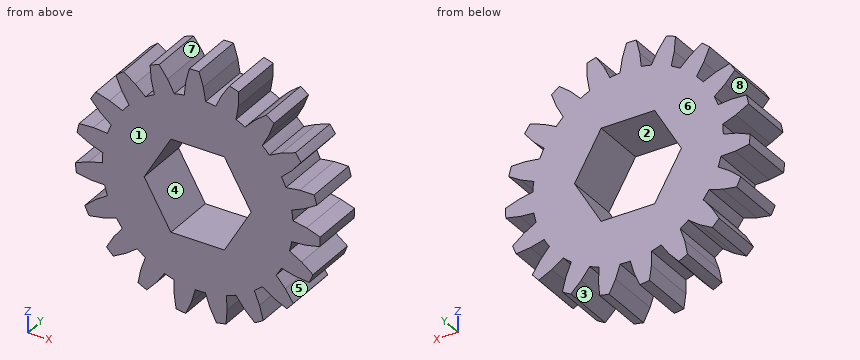
```python
from build123d import *

# Parameters (mm, degrees)
BOSS_EXTRUDE1_DEPTH      = 2.5
BOSS_EXTRUDE1_DEPTH_BACK = 2.5
SKETCH3_R                = 11.25
CUT_EXTRUDE1_DEPTH       = 17.105123408
CUT_EXTRUDE1_DEPTH_BACK  = 17.105123408
CUT_EXTRUDE2_DEPTH       = 17.676263216


with BuildPart() as part:
    # Sketch3 → Boss-Extrude1 (new, two sides: drawn at the far end of the back side and taken through both)
    with BuildSketch(Plane(origin=(0, 0, 0), x_dir=(1, 0, 0), z_dir=(0, 1, 0)).offset(-BOSS_EXTRUDE1_DEPTH_BACK)):
        with Locations(Location((0, 0, 0), (0, 0, 270))):
            Circle(SKETCH3_R)
    extrude(amount=BOSS_EXTRUDE1_DEPTH + BOSS_EXTRUDE1_DEPTH_BACK)

    # Sketch1 → Cut-Extrude1 (cut, two sides: drawn at the far end of the back side and taken through both)
    with BuildSketch(Plane(origin=(0, 0, 0), x_dir=(1, 0, 0), z_dir=(0, 1, 0)).offset(-CUT_EXTRUDE1_DEPTH_BACK)):
        with BuildLine():
            Line((1.131858911, 9.935738292), (0.713336296, 8.720874459))
            ThreePointArc((0.713336296, 8.720874459), (0.24791183, 8.746487279), (-0.218216182, 8.747278531))
            Line((-0.218216182, 8.747278531), (-0.567253557, 9.983898207))
            Line((-0.567253557, 9.983898207), (-1.093414937, 11.196738086))
            ThreePointArc((-1.093414937, 11.196738086), (0.318743782, 11.245483645), (1.725874204, 11.116827705))
            Line((1.725874204, 11.116827705), (1.131858911, 9.935738292))
        make_face()
        with BuildLine():
            Line((4.296660623, 9.029878598), (3.506349076, 8.016733509))
            ThreePointArc((3.506349076, 8.016733509), (3.074459061, 8.192081633), (2.633844069, 8.344181531))
            Line((2.633844069, 8.344181531), (2.705248253, 9.627129992))
            Line((2.705248253, 9.627129992), (2.601404214, 10.945099182))
            ThreePointArc((2.601404214, 10.945099182), (3.952875935, 10.532676386), (5.241989634, 9.954096879))
            Line((5.241989634, 9.954096879), (4.296660623, 9.029878598))
        make_face()
        with BuildLine():
            Line((6.995852487, 7.145491445), (5.919394526, 6.443855092))
            ThreePointArc((5.919394526, 6.443855092), (5.567840946, 6.749936829), (5.200486446, 7.036862989))
            Line((5.200486446, 7.036862989), (5.684594439, 8.227112863))
            Line((5.684594439, 8.227112863), (6.014320853, 9.507388951))
            ThreePointArc((6.014320853, 9.507388951), (7.158652645, 8.678490209), (8.19005415, 7.712685202))
            Line((8.19005415, 7.712685202), (6.995852487, 7.145491445))
        make_face()
        with BuildLine():
            Line((8.936935181, 4.48677942), (7.690981731, 4.172684988))
            ThreePointArc((7.690981731, 4.172684988), (7.457860872, 4.576331633), (7.203575423, 4.966991153))
            Line((7.203575423, 4.966991153), (8.047926613, 5.935560398))
            Line((8.047926613, 5.935560398), (8.775492506, 7.039405605))
            ThreePointArc((8.775492506, 7.039405605), (9.588678264, 5.883854957), (10.250599217, 4.635484408))
            Line((10.250599217, 4.635484408), (8.936935181, 4.48677942))
        make_face()
        with BuildLine():
            Line((9.909562279, 1.341855225), (8.629131728, 1.44933972))
            ThreePointArc((8.629131728, 1.44933972), (8.539705851, 1.906809896), (8.426045228, 2.358868756))
            Line((8.426045228, 2.358868756), (9.539141061, 3.000797864))
            Line((9.539141061, 3.000797864), (10.58570338, 3.808593434))
            ThreePointArc((10.58570338, 3.808593434), (10.979621808, 2.451612724), (11.200332804, 1.055956952))
            Line((11.200332804, 1.055956952), (9.909562279, 1.341855225))
        make_face()
        with BuildLine():
            Line((9.80833454, -1.948479804), (8.632181407, -1.431063996))
            ThreePointArc((8.632181407, -1.431063996), (8.696141194, -0.96934428), (8.735422289, -0.504873673))
            Line((8.735422289, -0.504873673), (9.99664156, -0.25914768))
            Line((9.99664156, -0.25914768), (11.248789039, 0.165061068))
            ThreePointArc((11.248789039, 0.165061068), (11.180752964, -1.246299789), (10.936336541, -2.637999824))
            Line((10.936336541, -2.637999824), (9.80833454, -1.948479804))
        make_face()
        with BuildLine():
            Line((8.644221562, -5.027666813), (7.699800288, -4.156389722))
            ThreePointArc((7.699800288, -4.156389722), (7.910214704, -3.740454963), (8.098180801, -3.313905205))
            Line((8.098180801, -3.313905205), (9.370850832, -3.491010552))
            Line((9.370850832, -3.491010552), (10.692893862, -3.496358227))
            ThreePointArc((10.692893862, -3.496358227), (10.170276048, -4.809156382), (9.487218518, -6.046088387))
            Line((9.487218518, -6.046088387), (8.644221562, -5.027666813))
        make_face()
        with BuildLine():
            Line((6.543373049, -7.56202811), (5.933026334, -6.431306129))
            ThreePointArc((5.933026334, -6.431306129), (6.267093712, -6.106229312), (6.583375767, -5.763823688))
            Line((6.583375767, -5.763823688), (7.729583013, -6.344568263))
            Line((7.729583013, -6.344568263), (8.978257718, -6.778892855))
            ThreePointArc((8.978257718, -6.778892855), (8.057691915, -7.850866258), (7.01001316, -8.798989458))
            Line((7.01001316, -8.798989458), (6.543373049, -7.56202811))
        make_face()
        with BuildLine():
            Line((3.733448535, -9.276926325), (3.523316916, -8.009290725))
            ThreePointArc((3.523316916, -8.009290725), (3.944835871, -7.810298967), (4.355159817, -7.58914244))
            Line((4.355159817, -7.58914244), (5.250694938, -8.510593556))
            Line((5.250694938, -8.510593556), (6.290688039, -9.326829258))
            ThreePointArc((6.290688039, -9.326829258), (5.071931835, -10.041812957), (3.773164105, -10.598383492))
            Line((3.773164105, -10.598383492), (3.733448535, -9.276926325))
        make_face()
        with BuildLine():
            Line((0.518946942, -9.986525626), (0.73180144, -8.719344394))
            ThreePointArc((0.73180144, -8.719344394), (1.195093854, -8.668001539), (1.654994723, -8.59205985))
            Line((1.654994723, -8.59205985), (2.202812593, -9.754363981))
            Line((2.202812593, -9.754363981), (2.9214247, -10.864058989))
            ThreePointArc((2.9214247, -10.864058989), (1.536549241, -11.144573407), (0.127434172, -11.249278223))
            Line((0.127434172, -11.249278223), (0.518946942, -9.986525626))
        make_face()
        with BuildLine():
            Line((-2.751790604, -9.613929918), (-2.139016077, -8.484521803))
            ThreePointArc((-2.139016077, -8.484521803), (-1.684155126, -8.586391647), (-1.224514728, -8.663894256))
            Line((-1.224514728, -8.663894256), (-1.083778676, -9.941097715))
            Line((-1.083778676, -9.941097715), (-0.764420336, -11.223999356))
            ThreePointArc((-0.764420336, -11.223999356), (-2.165342305, -11.039646403), (-3.532105231, -10.681139108))
            Line((-3.532105231, -10.681139108), (-2.751790604, -9.613929918))
        make_face()
        with BuildLine():
            Line((-5.72432894, -8.199515729), (-4.778038012, -7.330269624))
            ThreePointArc((-4.778038012, -7.330269624), (-4.380899766, -7.574312988), (-3.971329009, -7.796861285))
            Line((-3.971329009, -7.796861285), (-4.25292571, -9.050559259))
            Line((-4.25292571, -9.050559259), (-4.367428567, -10.367645235))
            ThreePointArc((-4.367428567, -10.367645235), (-5.632585414, -9.738402413), (-6.808886226, -8.955532836))
            Line((-6.808886226, -8.955532836), (-5.72432894, -8.199515729))
        make_face()
        with BuildLine():
            Line((-8.076547414, -5.896556781), (-6.899285389, -5.38166899))
            ThreePointArc((-6.899285389, -5.38166899), (-6.60290594, -5.741439989), (-6.28778817, -6.084917413))
            Line((-6.28778817, -6.084917413), (-6.961202251, -7.179252274))
            Line((-6.961202251, -7.179252274), (-7.497158145, -8.387795881))
            ThreePointArc((-7.497158145, -8.387795881), (-8.489450494, -7.381851415), (-9.347818747, -6.259455621))
            Line((-9.347818747, -6.259455621), (-8.076547414, -5.896556781))
        make_face()
        with BuildLine():
            Line((-9.553546654, -2.954614412), (-8.272888141, -2.849881016))
            ThreePointArc((-8.272888141, -2.849881016), (-8.1093848, -3.28639288), (-7.922867918, -3.713578323))
            Line((-7.922867918, -3.713578323), (-8.915124515, -4.529961907))
            Line((-8.915124515, -4.529961907), (-9.814454308, -5.498998694))
            ThreePointArc((-9.814454308, -5.498998694), (-10.426351886, -4.225362275), (-10.873770061, -2.885069265))
            Line((-10.873770061, -2.885069265), (-9.553546654, -2.954614412))
        make_face()
        with BuildLine():
            Line((-9.995270876, 0.307506274), (-8.749995096, -0.009264214))
            ThreePointArc((-8.749995096, -0.009264214), (-8.737085987, -0.475214109), (-8.69938199, -0.939815399))
            Line((-8.69938199, -0.939815399), (-9.902954705, -1.389779878))
            Line((-9.902954705, -1.389779878), (-11.068202059, -2.014299673))
            ThreePointArc((-11.068202059, -2.014299673), (-11.233396269, -0.610989569), (-11.221379665, 0.801959113))
            Line((-11.221379665, 0.801959113), (-9.995270876, 0.307506274))
        make_face()
        with BuildLine():
            Line((-9.353852406, 3.536303884), (-8.278904312, 2.83235651))
            ThreePointArc((-8.278904312, 2.83235651), (-8.417988338, 2.387461485), (-8.53318304, 1.935791107))
            Line((-8.53318304, 1.935791107), (-9.817646093, 1.901006365))
            Line((-9.817646093, 1.901006365), (-11.122538377, 1.688679973))
            ThreePointArc((-11.122538377, 1.688679973), (-10.823127863, 3.069593338), (-10.352978664, 4.402082777))
            Line((-10.352978664, 4.402082777), (-9.353852406, 3.536303884))
        make_face()
        with BuildLine():
            Line((-7.698798888, 6.381888097), (-6.910665785, 5.367047457))
            ThreePointArc((-6.910665785, 5.367047457), (-7.186671034, 4.991418581), (-7.442281301, 4.601624609))
            Line((-7.442281301, 4.601624609), (-8.668443189, 4.985789072))
            Line((-8.668443189, 4.985789072), (-9.971575077, 5.208664942))
            ThreePointArc((-9.971575077, 5.208664942), (-9.240005615, 6.417538176), (-8.362671783, 7.525172467))
            Line((-8.362671783, 7.525172467), (-7.698798888, 6.381888097))
        make_face()
        with BuildLine():
            Line((-5.209461051, 8.535895709), (-4.79354939, 7.320135534))
            ThreePointArc((-4.79354939, 7.320135534), (-5.17656641, 7.054478025), (-5.544892904, 6.768800683))
            Line((-5.544892904, 6.768800683), (-6.579879962, 7.53028417))
            Line((-6.579879962, 7.53028417), (-7.740036893, 8.164210243))
            ThreePointArc((-7.740036893, 8.164210243), (-6.655585384, 9.070043175), (-5.466139653, 9.832792955))
            Line((-5.466139653, 9.832792955), (-5.209461051, 8.535895709))
        make_face()
        with BuildLine():
            Line((-2.155597276, 9.764906573), (-2.15697754, 8.479973343))
            ThreePointArc((-2.15697754, 8.479973343), (-2.605500493, 8.353075313), (-3.046629323, 8.202472174))
            Line((-3.046629323, 8.202472174), (-3.778284643, 9.258756134))
            Line((-3.778284643, 9.258756134), (-4.669745613, 10.235036683))
            ThreePointArc((-4.669745613, 10.235036683), (-3.349929206, 10.739668259), (-1.977266476, 11.074877755))
            Line((-1.977266476, 11.074877755), (-2.155597276, 9.764906573))
        make_face()
    extrude(amount=CUT_EXTRUDE1_DEPTH + CUT_EXTRUDE1_DEPTH_BACK, mode=Mode.SUBTRACT)

    # Sketch4 → Cut-Extrude2 (cut, through all)
    with BuildSketch(Plane(origin=(0, 2.5, 0), x_dir=(1, 0, 0), z_dir=(0, 1, 0))):
        Polygon((4.907477288, 0), (2.453738644, 4.25), (-2.453738644, 4.25), (-4.907477288, 0), (-2.453738644, -4.25), (2.453738644, -4.25), align=None)
    extrude(amount=-CUT_EXTRUDE2_DEPTH, mode=Mode.SUBTRACT)


solid = part.part
```
Geometry check sheet. Reference: the model listing, model coordinates, mm. Face numbers are marked on the shaded views. A direction names the side the tool comes from. Coordinates: 2 decimals unless noted, no trailing zeros. Order: outer loops, then holes, each group sorted by start corner. A loop starts at its lowest first (then second) coordinate and runs counter-clockwise, first axis right, second up.
Item 1: Mould release check, pull along Z, two halves, no side actions. Record for the marked faces 1, 2 and 3: released by +Z, released by -Z, zero draft, split by the parting line, or undercut.
Item 2: Depth check by flat-ended pin: pin 1 (3 mm diameter, centred on x = -2.5, y = -1, fed in from +Z); pin 2 (1 mm diameter, centred on x = -7, y = 0, fed in from +Z). Enter the tip coordinate at first touch or a pass-through.
Item 3: Tool access check on the marked faces 4, 5, 6, 7 and 8. Record the directions out of +Z, -Z, +X, -X, +Y, -Y that give a thin tool (end or side, any length) a straight path to the whole face; none if there is none.
Item 4: Section check A-A (x = -6). Enter the section's corners in (y, z).
Item 5: Scan lines: line 1 along Z through (x, y) = (2, 2.15); line 2 along Z through (x, y) = (-10, 2.3); line 3 along X through (y, z) = (1.65, -3.5). Record each from-to range of solid material in increasing order.
Check sheet entries:
1. face 1: zero draft
1. face 2: undercut
1. face 3: released by -Z
2. pin 1: stops at z = 10.68
2. pin 2: stops at z = 8.96
3. face 4: +Y, -Y
3. face 5: +X, +Y, -Y
3. face 6: +Z, -Z, +X, -X, +Y
3. face 7: +Z, +Y, -Y
3. face 8: -X, +Y, -Y
4. outline: (-2.5, -7.1) - (2.5, -7.1) - (2.5, 8.39) - (-2.5, 8.39) - close
5. line 1: z = -11.07 to -4.25, 4.25 to 9.32
5. line 2: z = -5.15 to -4.1, -1.87 to -0.31, 1.44 to 2.93
5. line 3: x = -9.3 to -2.89, 2.89 to 10.19
